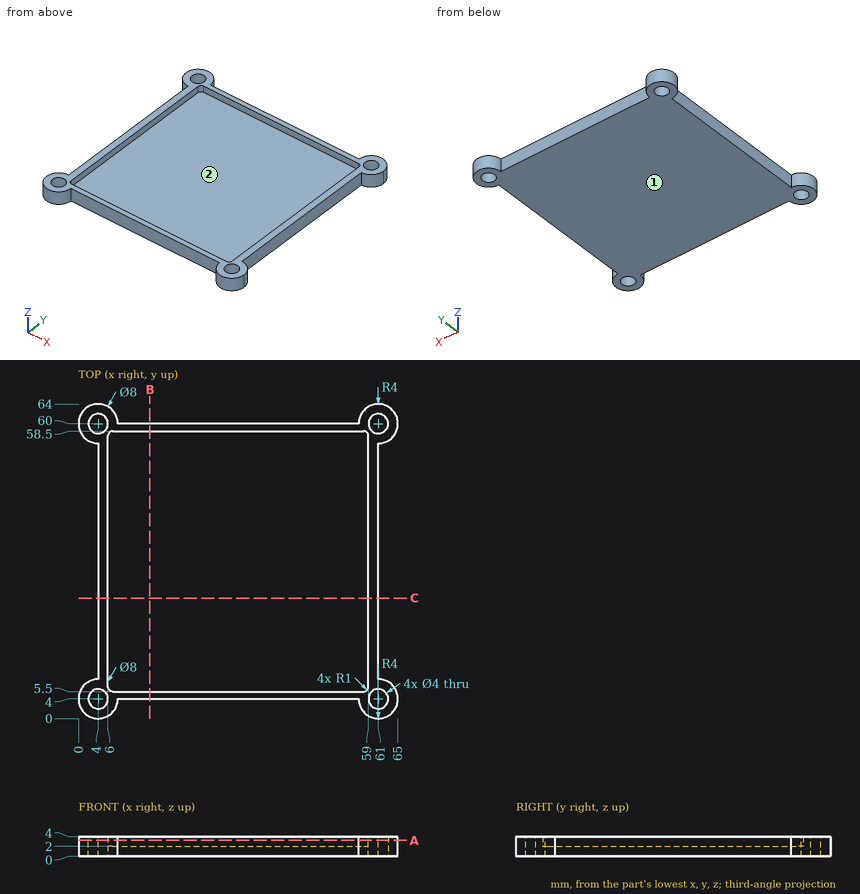
Job drawing, mm, ordinate dimensions from the low corner. One solid piece. Round coordinates to 2 decimals unless told otherwise and drop trailing zeros. Loops run counter-clockwise (first coordinate to the right, second up) from the corner with the lowest first, then second, coordinate; pieces in that order, holes last.
Item 1: Drop flat-ended pins along their axis: P1, Ø0.6, axis at y = 22, z = 2.5, coming from the -X side; P2, Ø16, axis at x = 43.5, y = 41, coming from the +Z side; P3, Ø1, axis at x = 41, z = 2.5, coming from the -Y side; P4, Ø3.5, axis at x = 4, y = 60, coming from the +Z side. Give the stop position or say it passes through.
Item 2: Cut at A-A, the plane z = 3.2. Give the cut face in (x, y), then the cut area to 3 significant figures.
Item 3: Cut at C-C, the plane y = 24.5. Give the cut face in (x, z), then the cut area to 3 significant figures.
Item 4: Drill centre lines: line 1 (X direction, y = 41, z = 3.5); line 2 (Y direction, x = 14, z = 2.4); line 3 (Z direction, x = 16, y = 10). Where is each one in solid material? Low to high.
Item 5: Mould opens along X. For the marked faces 1 and 2 say: +X half, -X half, draft (parallel to the pull), parting line (faces both ways), or undercut.
Item 6: Cut at B-B, the plane x = 14.5. Give the cut face in (y, z).
A:
1. P1: stops at x = 4
1. P2: stops at z = 2
1. P3: stops at y = 4
1. P4: passes through
2. outline: (4, 8) arc R4 ccw (long way) to (8, 4) - (57, 4) arc R4 ccw (long way) to (61, 8) - (61, 56) arc R4 ccw (long way) to (57, 60) - (8, 60) arc R4 ccw (long way) to (4, 56) - close; hole circle Ø4 at (4, 4); hole circle Ø4 at (4, 60); hole (6, 6.5) arc R1 ccw to (7, 5.5) - (58, 5.5) arc R1 ccw to (59, 6.5) - (59, 57.5) arc R1 ccw to (58, 58.5) - (7, 58.5) arc R1 ccw to (6, 57.5) - close; hole circle Ø4 at (61, 4); hole circle Ø4 at (61, 60)
2. area: 484 mm2
3. outline: (4, 0) - (61, 0) - (61, 4) - (59, 4) - (59, 2) - (6, 2) - (6, 4) - (4, 4) - close
3. area: 122 mm2
4. line 1: x = 4 to 6, 59 to 61
4. line 2: y = 4 to 5.5, 58.5 to 60
4. line 3: z = 0 to 2
5. face 1: draft
5. face 2: undercut
6. outline: (4, 0) - (60, 0) - (60, 4) - (58.5, 4) - (58.5, 2) - (5.5, 2) - (5.5, 4) - (4, 4) - close
